Read the model definition and answer for the solid it produces. Units are mm, in the model's axes. A direction names the side the tool comes from. Coordinates: 2 decimals unless noted, no trailing zeros. Order: outer loops, then holes, each group sorted by start corner. A loop starts at its lowest first (then second) coordinate and runs counter-clockwise, first axis right, second up. Notation, with made-up numbers: (2, -40) -> (9, -40) arc R18 ccw to (9, -32) -> close; hole circle Ø9 at (15, -12). An arc over 180 degrees is marked (long way). Answer as a JSON object with one key per item and string values. Group by question number.
1) Section D-D on x = 2 is taken. Determine the outline of the cut face in (y, z).
2) Section A-A on x = -56.25 is taken. Determine the outline of the cut face in (y, z).
3) Section B-B on z = -30 is taken. Determine the outline of the cut face in (x, y) (3 decimals), and give its area (3 significant figures).
4) Given pin 1 (7.5 mm diameter, centred on y = 10.5, z = -9.5, fed in from +X); pin 2 (1.5 mm diameter, centred on x = -24, z = -35.5, fed in from +Y); pin 3 (5 mm diameter, centred on y = -8, z = -44.5, fed in from +X), each flat-ended and moving along its own axis, determine where each tip first touches the part or whether it passes through.
5) Consider L1, parallel to Y at x = -56, z = -5; L2, parallel to Z at x = -54, y = 44; L3, parallel to Z at x = -22.5, y = -17.5. Determine where each line is inside the solid, lowest interval first.
6) Determine the mould class of faces 6 (the cylindrical face through (-64.19, 23.92, -7.4)), 7 (the flat face through (-56.51, 19.85, -15)), 8 (the flat face through (-37.5, 16, -52)), 9 (the cylindrical face through (-24.37, -14.79, -30.33)) for opening direction X: released by +X, released by -X, zero draft, split by the parting line, or undercut.
7) A tool of negligible diameter and unlimited length cuts with its end or side. For faces 1 (the flat face through (-37.5, 16, -7)), 2 (the cylindrical face through (-64.19, 23.92, -52.4)), 3 (the flat face through (-1, 0, -50)), 4 (the flat face through (19, -15, -45)), 5 (the flat face through (-56.51, 19.85, -45)), from which of +Z, -Z, +X, -X, +Y, -Y can it reach the whole face along a straight path? Write none if from no direction.
8) Section C-C on y = 28 is taken. Determine the outline of the cut face in (x, z), and give its area (3 significant figures).
from build123d import *

# Parameters (mm, degrees)
SKETCH1_R           = 10
BOSS_EXTRUDE1_DEPTH = 60
SKETCH3_W           = 37.5
SKETCH3_H           = 30
CUT_EXTRUDE1_DEPTH  = 108.710549623
CUT_EXTRUDE2_DEPTH  = 108.710549623
FILLET1_RADIUS      = 30
FILLET1_LENGTH      = 30
FILLET2_R           = 2


with BuildPart() as part:
    # Sketch1 → Boss-Extrude1 (new body)
    with BuildSketch(Plane.XY):
        with BuildLine():
            Line((75, 0), (75, -30))
            Line((75, -30), (-75, -30))
            Line((-75, -30), (-75, 30))
            ThreePointArc((-75, 30), (-56.25, 48.75), (-37.5, 30))
            Line((-37.5, 30), (-37.5, 0))
            Line((-37.5, 0), (75, 0))
        make_face()
        with Locations((-56.25, 30)):
            Circle(SKETCH1_R, mode=Mode.SUBTRACT)
    extrude(amount=-BOSS_EXTRUDE1_DEPTH)

    # Sketch3 → Cut-Extrude1 (cut, through all)
    with BuildSketch(Plane(origin=(0, 0, 0), x_dir=(1, 0, 0), z_dir=(0, 1, 0))):
        with Locations((-56.25, 30)):
            Rectangle(SKETCH3_W, SKETCH3_H)
    extrude(amount=CUT_EXTRUDE1_DEPTH, mode=Mode.SUBTRACT)

    # Sketch3<5> → Cut-Extrude2 (cut, through all)
    with BuildSketch(Plane(origin=(0, 0, 0), x_dir=(1, 0, 0), z_dir=(0, 1, 0))):
        with BuildLine():
            Line((46.875, 45), (-9.375, 45))
            ThreePointArc((-9.375, 45), (-24.375, 30), (-9.375, 15))
            Line((-9.375, 15), (46.875, 15))
            ThreePointArc((46.875, 15), (61.875, 30), (46.875, 45))
        make_face()
    extrude(amount=-CUT_EXTRUDE2_DEPTH, mode=Mode.SUBTRACT)

    # Fillet1: full round fillet: the end face becomes a half cylinder, R = half its width
    fillet1_face = Plane((75, -15, -30), x_dir=(0, 1, 0), z_dir=(1, 0, 0))  # on the end face: x along it, z out of the body
    fillet1_slab = fillet1_face.offset(-FILLET1_RADIUS / 2) * Box(FILLET1_LENGTH, 2 * FILLET1_RADIUS, FILLET1_RADIUS, mode=Mode.PRIVATE)  # the body's end, R deep
    fillet1_round = Plane((45, -15, -30), x_dir=(1, 0, 0), z_dir=(0, 1, 0)) * Cylinder(FILLET1_RADIUS, FILLET1_LENGTH, mode=Mode.PRIVATE)  # its axis R under the face
    add(fillet1_slab - fillet1_round, mode=Mode.SUBTRACT)

    # Fillet2
    fillet2_edges = [part.edges().sort_by_distance(p)[0] for p in [
        (-37.5, 0, -52.5),
        (-37.5, 0, -7.5),
        (-56.25, 0, -45),
        (-56.25, 0, -15),
    ]]
    fillet(fillet2_edges, radius=FILLET2_R)


solid = part.part
Worked answers:
{
 "1": {"outline": "(-30, -60) -> (0, -60) -> (0, -45) -> (-30, -45) -> close; (-30, -15) -> (0, -15) -> (0, 0) -> (-30, 0) -> close"},
 "2": {"outline": "(-30, -60) -> (20, -60) -> (20, -45) -> (2, -45) arc R2 cw to (0, -43) -> (0, -17) arc R2 cw to (2, -15) -> (20, -15) -> (20, 0) -> (-30, 0) -> close; (40, -60) -> (48.75, -60) -> (48.75, -45) -> (40, -45) -> close; (40, -15) -> (48.75, -15) -> (48.75, 0) -> (40, 0) -> close"},
 "3": {"outline": "(-75, -30) -> (-24.375, -30) -> (-24.375, 0) -> (-75, 0) -> close; (61.875, -30) -> (75, -30) -> (75, 0) -> (61.875, 0) -> close", "area": "1,910 mm²"},
 "4": {"pin 1": "stops at x = -37.5", "pin 2": "stops at y = 0", "pin 3": "stops at x = 72.5"},
 "5": {"L1": "y = -30 to 20, 40 to 48.75", "L2": "z = -60 to -45, -15 to 0", "L3": "z = -60 to -37.26, -22.74 to 0"},
 "6": {"face 6": "undercut", "face 7": "zero draft", "face 8": "released by +X", "face 9": "undercut"},
 "7": {"face 1": "+Z, -Z, +X, +Y", "face 2": "+Z, -Z", "face 3": "+X, +Y", "face 4": "+Y, -Y", "face 5": "+X, -X, +Y"},
 "8": {"outline": "(-75, -60) -> (-66.05, -60) -> (-66.05, -45) -> (-75, -45) -> close; (-75, -15) -> (-66.05, -15) -> (-66.05, 0) -> (-75, 0) -> close; (-46.45, -60) -> (-37.5, -60) -> (-37.5, -45) -> (-46.45, -45) -> close; (-46.45, -15) -> (-37.5, -15) -> (-37.5, 0) -> (-46.45, 0) -> close", "area": "537 mm²"}
}
